Check sheet for the modelled part. Datum: model origin and axes. Units: mm. Coordinates: 2 decimals unless noted, no trailing zeros. Loops run counter-clockwise (first coordinate to the right, second up) from the corner with the lowest first, then second, coordinate; pieces in that order, holes last. Notation, with made-up numbers: (13, 2) -> (38, 2) arc R14 ccw to (38, 17) -> close; hole circle Ø2 at (-3.5, 44). An arc over 180 degrees is marked (long way). Use CSV: the item, a comma, the result in double quotes. Start each with the question number.
1. Thickness scan on L1, parallel to Y at x = 0, z = 4.75; L2, parallel to Z at x = 9, y = 14; L3, parallel to Y at x = 3.5, z = 10.25. Record the ranges inside material, lowest first.
2. Sectioned sample at C-C, the plane x = -3. Record the cut outline in (y, z), and give its area (3 significant figures).
3. Gauge pin test, flat ends, axial feed: pin 1 (1 mm diameter, centred on x = -11.5, z = 4.5, fed in from -Y); pin 2 (10 mm diameter, centred on x = -4, z = 3.5, fed in from +Y); pin 3 (2 mm diameter, centred on x = -9, z = 9.5, fed in from +Y). Record the tip position at first contact, or that the pin passes through.
4. Sectioned sample at D-D, the plane z = 20.5. Record the cut outline in (x, y).
5. Sectioned sample at B-B, the plane y = -14.5. Record the cut outline in (x, z), and give its area (3 significant figures).
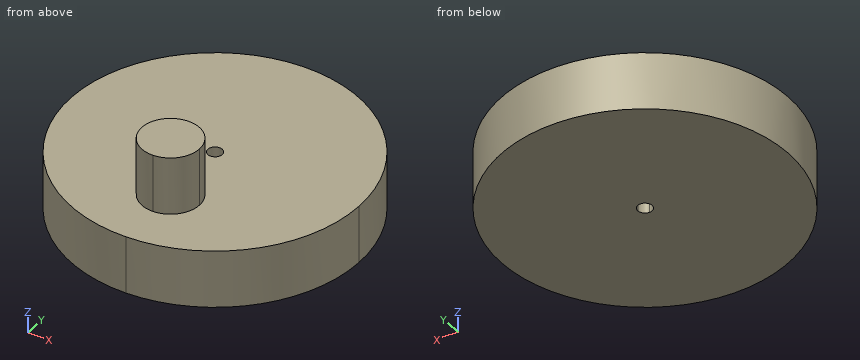
```python
from build123d import *

# Parameters (mm, degrees)
F1_DEPTH = 12.7
F2_DEPTH = 25.4


with BuildPart() as f1:
    # F0 (on Top) → F1 (new body)
    with BuildSketch(Plane.XY):
        with BuildLine():
            ThreePointArc((1.5875, 0), (-1.144027, 1.100617), (0.061379, -1.586313))
            ThreePointArc((0.061379, -1.586313), (1.144027, -1.100617), (1.5875, 0))
        make_face()
        with BuildLine():
            ThreePointArc((1.227574, -31.72626), (22.880537, -22.012349), (31.75, 0))
            ThreePointArc((31.75, 0), (-22.880537, 22.012349), (1.227574, -31.72626))
        make_face()
        with BuildLine():
            ThreePointArc((6.963787, -15.86313), (5.189894, -20.2656), (0.859301, -22.208382))
            ThreePointArc((0.859301, -22.208382), (-5.731465, -16.108645), (0.368272, -9.517878))
            ThreePointArc((0.368272, -9.517878), (5.016257, -11.287022), (6.963787, -15.86313))
        make_face(mode=Mode.SUBTRACT)
        with BuildLine():
            ThreePointArc((1.5875, 0), (1.144027, -1.100617), (0.061379, -1.586313))
            ThreePointArc((0.061379, -1.586313), (-1.144027, 1.100617), (1.5875, 0))
        make_face(mode=Mode.SUBTRACT)
    extrude(amount=F1_DEPTH)

    # F0 (on Top) → F2 (join)
    with BuildSketch(Plane.XY):
        with BuildLine():
            Line((0.368272, -9.517878), (0.859301, -22.208382))
            ThreePointArc((0.859301, -22.208382), (5.189894, -20.2656), (6.963787, -15.86313))
            ThreePointArc((6.963787, -15.86313), (5.016257, -11.287022), (0.368272, -9.517878))
        make_face()
        with BuildLine():
            ThreePointArc((0.368272, -9.517878), (-5.731465, -16.108645), (0.859301, -22.208382))
            Line((0.859301, -22.208382), (0.368272, -9.517878))
        make_face()
    extrude(amount=F2_DEPTH)


solid = f1.part
```
Completed:
1,L1,"-31.75 to -1.59, 1.59 to 31.75"
1,L2,"0 to 12.7"
1,L3,"-31.56 to 31.56"
2,outline,"(-31.61, 0) -> (31.61, 0) -> (31.61, 12.7) -> (-10.64, 12.7) -> (-10.64, 25.4) -> (-21.08, 25.4) -> (-21.08, 12.7) -> (-31.61, 12.7) -> close"
2,area,"935 mm²"
3,pin 1,"y = -29.78"
3,pin 2,"y = 31.75"
3,pin 3,"y = 30.73"
4,outline,"(0.37, -9.52) arc R6.35 ccw (long way) to (6.96, -15.86) arc R6.35 ccw to start"
5,outline,"(-28.25, 0) -> (28.25, 0) -> (28.25, 12.7) -> (6.82, 12.7) -> (6.82, 25.4) -> (-5.59, 25.4) -> (-5.59, 12.7) -> (-28.25, 12.7) -> close"
5,area,"875 mm²"
